Part model, mm, in its own coordinate system. A direction names the side the tool comes from. Round coordinates to 2 decimals unless told otherwise and drop trailing zeros. Loops run counter-clockwise (first coordinate to the right, second up) from the corner with the lowest first, then second, coordinate; pieces in that order, holes last. Notation, with made-up numbers: M 15,-18.5 L 40,-18.5 A12 cw 40,4.5 Z; hole C 37.5,-31.75 d6. An arc over 180 degrees is marked long. Write each question's results on one line, items separated by ' | '.
from build123d import *

# Parameters (mm, degrees)
F0_R           = 31.75
F1_DEPTH       = 6.35
F3_D           = 6.35
F3_CBORE_D     = 12.7
F3_CBORE_DEPTH = 6.35
F4_SIZE        = 1.524


with BuildPart() as f1:
    # F0 (on Front) → F1 (new body, symmetric)
    with BuildSketch(Plane.XZ):
        Circle(F0_R)
    extrude(amount=F1_DEPTH, both=True)

    # F3 (through all)
    with Locations(Plane.XZ.offset(6.35)):
        with Locations((-19.05, 10.998523), (0, 21.997045), (19.05, 10.998523), (19.05, -10.998523), (0, -21.997045), (-19.05, -10.998523)):
            CounterBoreHole(F3_D / 2, F3_CBORE_D / 2, F3_CBORE_DEPTH)

    # F4
    f4_edges = [f1.edges().sort_by_distance(p)[0] for p in [
        (-31.75, -6.35, 0),
    ]]
    chamfer(f4_edges, length=F4_SIZE)


solid = f1.part
Item 1: Band-saw the part on C-C on z = -9. Count the separate pieces of the cut face and the enclosed holes in it, and give its area (3 significant figures).
Filled sheet:
separate pieces: 3 | enclosed holes: 0 | area: 555 mm^2
Item 2: Which spindle directions (+Z, -Z, +X, -X, +Y, -Y) get a long thin tool onto all of the face, cutting with end or side? Do faces 3 (the cylindrical face through (0.688, 3.219, -25.097)), 4 (the flat face through (-21, 0, -8)). Say none if no direction does.
Filled sheet:
face 3: +Y, -Y | face 4: -Y
Item 3: Two-plate mould, pull along Z, no slides. Class faces 1 (the cylindrical face through (-24.089, -3.219, 7.135)), 2 (the flat face through (0, -6.35, 0)): +Z half, -Z half, draft (parallel to the pull), parting line (faces both ways), or undercut.
Filled sheet:
face 1: undercut | face 2: draft
Item 4: Band-saw the part on B-B on y = 4.25. Give the cut face in (x, z) (3 decimals), and give its area (3 significant figures).
Filled sheet:
outline: C 0,0 d63.5; hole C -19.05,-10.999 d6.35; hole C -19.05,10.999 d6.35; hole C 0,-21.997 d6.35; hole C 0,21.997 d6.35; hole C 19.05,-10.999 d6.35; hole C 19.05,10.999 d6.35 | area: 2,980 mm^2
Item 5: Band-saw the part on D-D on y = -1.5. Give the cut face in (x, z), and give its area (3 significant figures).
Filled sheet:
outline: C 0,0 d63.5; hole C -19.05,-11 d12.7; hole C -19.05,11 d12.7; hole C 0,-22 d12.7; hole C 0,22 d12.7; hole C 19.05,-11 d12.7; hole C 19.05,11 d12.7 | area: 2,410 mm^2
Item 6: Band-saw the part on A-A on x = 0. Give the cut face in (y, z), and give its area (3 significant figures).
Filled sheet:
outline: M -6.35,-30.23 L -4.83,-31.75 L 6.35,-31.75 L 6.35,-25.17 L 0,-25.17 L 0,-28.35 L -6.35,-28.35 Z; M -6.35,-15.65 L 0,-15.65 L 0,-18.82 L 6.35,-18.82 L 6.35,18.82 L 0,18.82 L 0,15.65 L -6.35,15.65 Z; M -6.35,28.35 L 0,28.35 L 0,25.17 L 6.35,25.17 L 6.35,31.75 L -4.83,31.75 L -6.35,30.23 Z | area: 562 mm^2
Item 7: Wall check: L1, parallel to Z at x = 19.05, y = -4.25; L2, parallel to Z at x = 19.05, y = 2.75; L3, parallel to X at y = -2.75, z = 7. Give the ranges that are in metal, low to high.
Filled sheet:
L1: -25.4 to -17.35, -4.65 to 4.65, 17.35 to 25.4 | L2: -25.4 to -14.17, -7.82 to 7.82, 14.17 to 25.4 | L3: -30.97 to -23.98, -14.12 to 14.12, 23.98 to 30.97
Item 8: Drop flat-ended pins along their axis: P1, Ø10, axis at x = -18.5, z = -8, coming from the -Y side; P2, Ø11.5, axis at x = -19.05, z = -11, coming from the -Y side; P3, Ø6, axis at x = -1, y = 3, coming from the +Z side; P4, Ø1.5, axis at x = -6, y = 0, coming from the +Z side. Give the stop position or say it passes through.
Filled sheet:
P1: y = -6.35 | P2: y = 0 | P3: z = 31.75 | P4: z = 31.31
